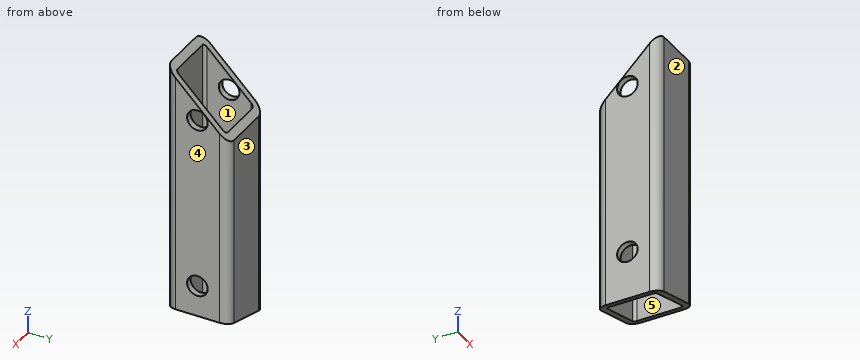
Autodesk Inventor part; units mm, degrees
ref_plane "Start Plane" through (0, 0, 7.6064) normal (0, 0, 1) x (1, 0, 0)
ref_plane "End Plane" through (0, 0, 93.0129) normal (0, 0, 1) x (1, 0, 0)
ref_plane "Work Plane4" through (4.0763, -100, 11.5058) normal (0.267, 0, -0.9637) x (-0.9637, 0, -0.267)
ref_plane "Start Plane" through (0, 0, 7.6064) normal (0, 0, 1) x (1, 0, 0)
ref_plane "End Plane" through (0, 0, 93.0129) normal (0, 0, 1) x (1, 0, 0)
sketch "Sketch" plane through (0, 0, 0) normal (0, 0, 1) x (1, 0, 0)
  line L0 (-10, -7) -> (-10, 7)
  line L1 (-7, 10) -> (7, 10)
  line L2 (10, 7) -> (10, -7)
  line L3 (7, -10) -> (-7, -10)
  arc A0 (-10, -7) -> (-7, -10) centre (-7, -7) ccw
  arc A1 (-7, 10) -> (-10, 7) centre (-7, 7) ccw
  arc A2 (10, 7) -> (7, 10) centre (7, 7) ccw
  arc A3 (7, -10) -> (10, -7) centre (7, -7) ccw
  arc A4 (-7, 8) -> (-8, 7) centre (-7, 7) ccw
  line L4 (-7, 8) -> (7, 8)
  arc A5 (8, 7) -> (7, 8) centre (7, 7) ccw
  line L5 (8, 7) -> (8, -7)
  arc A6 (7, -8) -> (8, -7) centre (7, -7) ccw
  line L6 (7, -8) -> (-7, -8)
  arc A7 (-8, -7) -> (-7, -8) centre (-7, -7) ccw
  line L7 (-8, -7) -> (-8, 7)
  line L8 (0, 14.8698) -> (0, -14.8698) construction
  line L9 (-14.8698, 0) -> (14.8698, 0) construction
  dimension "d7" = 3
  dimension "d10" = 20
  dimension "d11" = 20
  dimension "d12" = 2
  dimension "d15" = 10
  dimension "d16" = 10
extrude "Body" add sketch "Sketch" along normal up to surface (85.4065 mm away) from surface at 7.6064
sketch "Sketch3" plane through (0, 0, 0) normal (0, 0, 1) x (1, 0, 0)
  line L0 (0, 0) -> (10, 0)
ref_plane "Work Plane3" through (0, 0, 0) normal (0, -1, 0) x (1, 0, 0)
sketch "Sketch4" plane through (0, 0, 0) normal (0, -1, 0) x (1, 0, 0)
  line L0 (-2, 7.6064) -> (12, 7.6064)
  line L1 (-2, 93.0129) -> (12, 93.0129)
  dimension "d18" = 85.4065
ref_plane "Work Plane4" through (4.0763, -100, 11.5058) normal (0.267, 0, -0.9637) x (-0.9637, 0, -0.267)
split "Split1" plane through (4.0763, -100, 11.5058) removes the side toward (0.267, 0, -0.9637)
ref_plane "Work Plane6" through (0, -10, 93.0129) normal (0, 0.7071, 0.7071) x (1, 0, 0)
split "Split3" plane through (0, -10, 93.0129) removes the side toward (0, 0.7071, 0.7071)
sketch "Sketch7" plane through (8, -7, 12.5928) normal (-1, 0, 0) x (0, 0, 1)
  point P0 (10.554, 7)
hole "Hole3" at (8, 0, 23.1468) direction (1, 0, 0) diameter 6.6 depth 2
sketch "Sketch8" plane through (8, -7, 12.5928) normal (-1, 0, 0) x (0, 0, 1)
  point P0 (65.554, 7)
hole "Hole4" at (8, 0, 78.1468) direction (1, 0, 0) diameter 6.6 depth 2
sketch "Sketch9" plane through (-10, -7, 7.6064) normal (-1, 0, 0) x (0, 0, 1)
  point P0 (15.5404, 7)
hole "Hole5" at (-10, 0, 23.1468) direction (1, 0, 0) diameter 6.6 end through all
sketch "Sketch11" plane through (-10, -7, 7.6064) normal (-1, 0, 0) x (0, 0, 1)
  point P0 (70.5404, 7)
hole "Hole7" at (-10, 0, 78.1468) direction (1, 0, 0) diameter 6.6 end through all
equation "\"d7\" = G_IR"
equation "\"d10\" = G_H"
equation "\"d11\" = G_W"
equation "\"d12\" = G_T"
equation "\"d15\" = 0.5 * d10"
equation "\"d16\" = 0.5 * d11"
equation "\"d3\" = G_L"
equation "\"G_W\" = 20"
equation "\"G_H\" = 20"
equation "\"G_T\" = 2"
equation "\"G_IR\" = 3"
equation "\"G_L\" = d18"
equation "\"G_OFFSET_START\" = -7.60639"
equation "\"d13\" = -G_OFFSET_START"
equation "\"d14\" = G_OFFSET_END + B_L"
equation "\"B_L\" = 83.01292"
properties part number "ISO 12633-2 - 20x20x2 - 85,41" material "Steel, Mild"
Source: CAD feature listing. Evaluate the final solid. Frame: model axes, mm. Face numbers are marked on the shaded views. A direction names the side the tool comes from. Coordinates: 2 decimals unless noted, no trailing zeros. Order: outer loops, then holes, each group sorted by start corner. A loop starts at its lowest first (then second) coordinate and runs counter-clockwise, first axis right, second up. Notation, with made-up numbers: M -27.75,-22.5 L -12.75,-22.5 A11 ccw -12.75,-15.5 Z; hole C -30,64 d7. An arc over 180 degrees is marked long. Write each question's results on one line, items separated by ' | '. Start each with the question number.
1. Section B-B, the plane z = 57.5. Return the cut outline in (x, y).
2. Section C-C, the plane x = -1.5. Return the cut outline in (y, z).
3. Pin query (flat end, axial travel): pin 1 (4 mm diameter, centred on x = -7.5, y = 0, fed in from +Z). Return the tip coordinate at first contact, or that it passes through.
4. Section A-A, the plane y = 0. State how many separate pieces and enclosed holes the cut face has, then the cut area to 3 significant figures.
5. Reachability of the marked faces 1 and 2 from +Z, -Z, +X, -X, +Y, -Y: full face, straight path, thin tool, end or side. Return the list, or none.
6. Draft query along Y for the marked faces 3, 4 and 5. Return one class per face: +Y half, -Y half, draft (parallel to the pull), parting line (faces both ways), or undercut.
7. Material intervals for L1, parallel to Y at x = 3.5, z = 24.5; L2, parallel to Z at x = 8.9, y = 0, sorted ascending.
Solution:
1) outline: M -10,-7 A3 ccw -7,-10 L 7,-10 A3 ccw 10,-7 L 10,7 A3 ccw 7,10 L -7,10 A3 ccw -10,7 Z; hole M -8,-7 A1 ccw -7,-8 L 7,-8 A1 ccw 8,-7 L 8,7 A1 ccw 7,8 L -7,8 A1 ccw -8,7 Z
2) outline: M -10,9.96 L -8,9.96 L -8,91.01 L -10,93.01 Z; M 8,9.96 L 10,9.96 L 10,73.01 L 8,75.01 Z
3) pin 1: z = 84.95
4) separate pieces: 6 | enclosed holes: 0 | area: 238 mm²
5) face 1: +Z, -Z | face 2: +Z, -Z, +X, -X, -Y
6) face 3: +Y half | face 4: draft | face 5: undercut
7) L1: -10 to -8, 8 to 10 | L2: 12.84 to 19.85, 26.45 to 74.85, 81.45 to 83.01
